Model file for the job. Use its own axes, mm. Face numbers are marked on the shaded views. A direction names the side the tool comes from. Round coordinates to 2 decimals unless told otherwise and drop trailing zeros. Write each loop counter-clockwise with the first axis right and the second up, starting at its lowest first coordinate (ties: lowest second). Pieces come first, ordered by that corner, then holes. Notation, with made-up numbers: (-13, 37) - (0, 37) arc R23 ccw to (0, 52) - close; hole circle Ø2 at (-10.75, 59.5). An arc over 180 degrees is marked (long way). One line per item, written item: value.
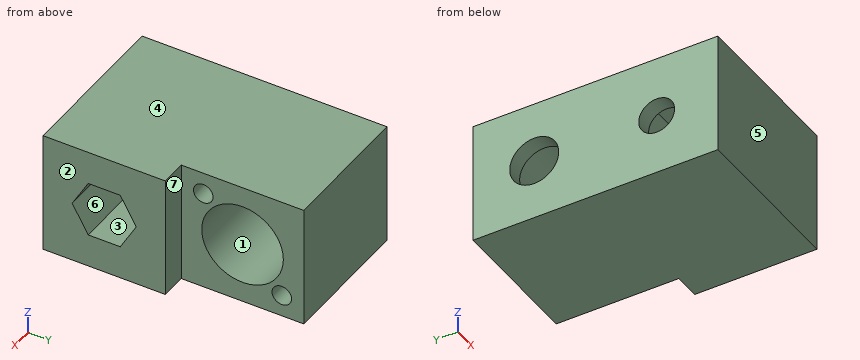
from build123d import *

# Parameters (mm, degrees)
F0_W     = 38.1
F0_H     = 19.05
F0_R     = 6.35
F1_DEPTH = 25.4
F2_W     = 38.1
F2_H     = 19.05
F2_R     = 3.81
F2_R_2   = 2.794
F3_DEPTH = 2.54
F4_W     = 19.05
F4_H     = 19.05
F5_DEPTH = 4.064
F6_R     = 1.524
F7_DEPTH = 19.05


with BuildPart() as f1:
    # F0 (on Right) → F1 (new body)
    with BuildSketch(Plane.YZ):
        Rectangle(F0_W, F0_H)
        Polygon((-14.510997, 0), (-12.017998, 4.318), (-7.032002, 4.318), (-4.539003, 0), (-7.032002, -4.318), (-12.017998, -4.318), align=None, mode=Mode.SUBTRACT)
        with Locations((9.525, 0)):
            Circle(F0_R, mode=Mode.SUBTRACT)
    extrude(amount=F1_DEPTH)

    # F2 (on face) → F3 (join)
    with BuildSketch(Plane(origin=(0, 0, 0), x_dir=(0, -1, 0), z_dir=(-1, 0, 0))):
        Rectangle(F2_W, F2_H)
        with Locations((-9.525, 0)):
            Circle(F2_R, mode=Mode.SUBTRACT)
        with Locations((9.525, 0)):
            Circle(F2_R_2, mode=Mode.SUBTRACT)
    extrude(amount=-F3_DEPTH)

    # F4 (on face) → F5 (cut)
    with BuildSketch(Plane.YZ.offset(25.4)):
        with Locations((9.525, 0)):
            Rectangle(F4_W, F4_H)
    extrude(amount=-F5_DEPTH, mode=Mode.SUBTRACT)

    # F6 (on face) → F7 (cut)
    with BuildSketch(Plane.YZ.offset(21.336)):
        with Locations((3.418426, 6.106574)):
            Circle(F6_R)
        with Locations((15.631574, -6.106574)):
            Circle(F6_R)
    extrude(amount=-F7_DEPTH, mode=Mode.SUBTRACT)


solid = f1.part
1. Band-saw the part on C-C on z = -1.25. Write the cut outline in (x, y), plus the area to 3 significant figures.
Report:
outline: (0, -19.05) - (25.4, -19.05) - (25.4, -13.79) - (2.54, -13.79) - (2.54, -12.02) - (0, -12.02) - close; (0, -7.03) - (2.54, -7.03) - (2.54, -5.26) - (25.4, -5.26) - (25.4, 0) - (21.34, 0) - (21.34, 3.3) - (2.54, 3.3) - (2.54, 5.93) - (0, 5.93) - close; (0, 13.12) - (2.54, 13.12) - (2.54, 15.75) - (21.34, 15.75) - (21.34, 19.05) - (0, 19.05) - close
area: 430 mm²
2. Band-saw the part on B-B on x = 12.25. Write the cut outline in (y, z) (3 decimals), plus the area to 3 significant figures.
Report:
outline: (-19.05, -9.525) - (19.05, -9.525) - (19.05, 9.525) - (-19.05, 9.525) - close; hole (-14.511, 0) - (-12.018, -4.318) - (-7.032, -4.318) - (-4.539, 0) - (-7.032, 4.318) - (-12.018, 4.318) - close; hole circle Ø3.048 at (3.418, 6.107); hole circle Ø12.7 at (9.525, 0); hole circle Ø3.048 at (15.632, -6.107)
area: 520 mm²
3. Band-saw the part on D-D on y = -13.5. Write the cut outline in (x, z) (3 decimals).
Report:
outline: (0, -9.525) - (25.4, -9.525) - (25.4, -1.751) - (2.54, -1.751) - (2.54, 1.751) - (25.4, 1.751) - (25.4, 9.525) - (0, 9.525) - close
4. Band-saw the part on A-A on y = -7.5. Write the cut outline in (x, z) (3 decimals), plus the area to 3 significant figures.
Report:
outline: (0, -9.525) - (25.4, -9.525) - (25.4, -4.318) - (2.54, -4.318) - (2.54, -1.925) - (0, -1.925) - close; (0, 1.925) - (2.54, 1.925) - (2.54, 4.318) - (25.4, 4.318) - (25.4, 9.525) - (0, 9.525) - close
area: 277 mm²
5. Mould opens along Z. For the marked faces 1, 2, 3 and 4 say: released by +Z, released by -Z, zero draft, split by the parting line, or undercut.
Report:
face 1: undercut
face 2: zero draft
face 3: undercut
face 4: released by +Z
6. Wall check: probe 1 along Y at (x, z) = (10.5, 1); probe 2 along Z at (x, y) = (6.75, -10) (3 decimals); probe 3 along Y at (x, z) = (18, 0.5). Give the ranges that are in metal, low to high. Write a range as [from, to].
Report:
probe 1: [-19.05, -13.93], [-5.12, 3.25], [15.8, 19.05]
probe 2: [-9.525, -4.318], [4.318, 9.525]
probe 3: [-19.05, -14.22], [-4.83, 3.19], [15.86, 19.05]
7. Drop flat-ended pins along their axis: pin 1 (9 mm diameter, centred on y = 9.525, z = 0, fed in from +X); pin 2 (2.5 mm diameter, centred on y = 3.42, z = 6.11, fed in from +X); pin 3 (3.5 mm diameter, centred on y = 2.5, z = 6, fed in from +X). Give the stop position or say it passes through.
Report:
pin 1: x = 2.54
pin 2: x = 2.29
pin 3: x = 21.34
8. Tool access for the marked faces 5, 6 and 7: list every direction of +Z, -Z, +X, -X, +Y, -Y with a clear straight run to the whole face (end or side of a thin tool).
Report:
face 5: +Z, -Z, +X, -X, -Y
face 6: +X
face 7: +Z, -Z, +X, +Y
